```python
from build123d import *

# Parameters (mm, degrees)
F0_W     = 79.3
F0_H     = 7.4
F0_R     = 3
F1_DEPTH = 3.95
F0_R_2   = 2.499
F2_DEPTH = 2.95
F3_R     = 3.69999


# Not quite as in the source:
# - a fillet or chamfer is up to 0.001 mm smaller than in the source, because OpenCascade refuses the exact size


with BuildPart() as f1:
    # F0 (on Front) → F1 (new body, symmetric)
    with BuildSketch(Plane.XZ):
        with Locations((-4, 0)):
            Rectangle(F0_W, F0_H)
        with Locations((-40, 0)):
            Circle(F0_R, mode=Mode.SUBTRACT)
        with Locations((-32, 0)):
            Circle(F0_R, mode=Mode.SUBTRACT)
        with Locations((-24, 0)):
            Circle(F0_R, mode=Mode.SUBTRACT)
        with Locations((-16, 0)):
            Circle(F0_R, mode=Mode.SUBTRACT)
        with Locations((-8, 0)):
            Circle(F0_R, mode=Mode.SUBTRACT)
        Circle(F0_R, mode=Mode.SUBTRACT)
        with Locations((8, 0)):
            Circle(F0_R, mode=Mode.SUBTRACT)
        with Locations((16, 0)):
            Circle(F0_R, mode=Mode.SUBTRACT)
        with Locations((24, 0)):
            Circle(F0_R, mode=Mode.SUBTRACT)
        with Locations((32, 0)):
            Circle(F0_R, mode=Mode.SUBTRACT)
    extrude(amount=F1_DEPTH, both=True)

    # F0 (on Front) → F2 (join, symmetric)
    with BuildSketch(Plane.XZ):
        with Locations((-40, 0)):
            Circle(F0_R)
        with Locations((-40, 0)):
            Circle(F0_R_2, mode=Mode.SUBTRACT)
        with Locations((-32, 0)):
            Circle(F0_R)
        with Locations((-32, 0)):
            Circle(F0_R_2, mode=Mode.SUBTRACT)
        with Locations((-24, 0)):
            Circle(F0_R)
        with Locations((-24, 0)):
            Circle(F0_R_2, mode=Mode.SUBTRACT)
        with Locations((-16, 0)):
            Circle(F0_R)
        with Locations((-16, 0)):
            Circle(F0_R_2, mode=Mode.SUBTRACT)
        with Locations((-8, 0)):
            Circle(F0_R)
        with Locations((-8, 0)):
            Circle(F0_R_2, mode=Mode.SUBTRACT)
        Circle(F0_R)
        Circle(F0_R_2, mode=Mode.SUBTRACT)
        with Locations((8, 0)):
            Circle(F0_R)
        with Locations((8, 0)):
            Circle(F0_R_2, mode=Mode.SUBTRACT)
        with Locations((16, 0)):
            Circle(F0_R)
        with Locations((16, 0)):
            Circle(F0_R_2, mode=Mode.SUBTRACT)
        with Locations((24, 0)):
            Circle(F0_R)
        with Locations((24, 0)):
            Circle(F0_R_2, mode=Mode.SUBTRACT)
        with Locations((32, 0)):
            Circle(F0_R)
        with Locations((32, 0)):
            Circle(F0_R_2, mode=Mode.SUBTRACT)
    extrude(amount=F2_DEPTH, both=True)

    # F3 (radius 3.7 in the source; OpenCascade refuses exactly that, so slightly less here)
    f3_edges = [f1.edges().sort_by_distance(p)[0] for p in [
        (-43.65, 0, 3.7),
        (35.65, 0, 3.7),
        (35.65, 0, -3.7),
        (-43.65, 0, -3.7),
    ]]
    fillet(f3_edges, radius=F3_R)


solid = f1.part
```
Read the model definition and answer for the solid it produces. Units are mm, in the model's axes. A direction names the side the tool comes from. Round coordinates to 2 decimals unless told otherwise and drop trailing zeros. Write each loop counter-clockwise with the first axis right and the second up, starting at its lowest first coordinate (ties: lowest second). Pieces come first, ordered by that corner, then holes. Notation, with made-up numbers: (-25, 89) -> (29, 89) arc R16 cw to (29, 119) -> close; hole circle Ø9 at (71, -0.75). An arc over 180 degrees is marked (long way). Answer in a Markdown table with one row per item. Add a question column.
1) Consider line 1 (Z direction, x = 0, y = -3.25); line 2 (Z direction, x = 0, y = -0.8). Determine where each line is inside the solid, lowest interval first.
2) Find section C-C, the plane x = 15. Determine the outline of the cut face in (y, z), and give its area (3 significant figures).
3) Determine the mould class of faces 1 (the face through (-4.6, -3.95, 0.1)), 2 (the face through (-42.59, -0.06, -2.59)), 3 (the face through (-3, -3.4, 0.1)) for opening direction X: pulls with the +X half, pulls with the -X half, needs draft (parallel to the pull), parting line crosses it, or undercut.
4) Given P1, Ø3, axis at x = 0, z = 0, coming from the +Y side; P2, Ø1.5, axis at y = 2.5, z = -1, coming from the +X side; P3, Ø2, axis at y = 1, z = -2, coming from the -X side; P4, Ø3, axis at x = -16.5, z = -1, coming from the +Y side, each flat-ended and moving along its own axis, determine where each tip first touches the part or whether it passes through.
5) Which of the six approach directions +Z, -Z, +X, -X, +Y, -Y give full straight-line access (tool end or side, diameter ignored) to faces 4 (the face through (-19, -3.4, 0.1)), 5 (the face through (13, 3.5, 0.1)), 6 (the face through (-4.6, 3.95, 0.1))?
6) Find section A-A, the plane x = -16. Determine the outline of the cut face in (y, z).
7) Find section B-B, the plane y = 1.75. State how many separate pieces and enclosed holes the cut face has, and give its area (3 significant figures).
Findings below:
| question | item | result |
|---|---|---|
| 1 | line 1 | -3.7 to -3, 3 to 3.7 |
| 1 | line 2 | -3.7 to -2.5, 2.5 to 3.7 |
| 2 | outline | (-3.95, -3.7) -> (3.95, -3.7) -> (3.95, -2.83) -> (2.95, -2.83) -> (2.95, -2.29) -> (-2.95, -2.29) -> (-2.95, -2.83) -> (-3.95, -2.83) -> close; (-3.95, 2.83) -> (-2.95, 2.83) -> (-2.95, 2.29) -> (2.95, 2.29) -> (2.95, 2.83) -> (3.95, 2.83) -> (3.95, 3.7) -> (-3.95, 3.7) -> close |
| 2 | area | 20.1 mm² |
| 3 | face 1 | needs draft |
| 3 | face 2 | pulls with the -X half |
| 3 | face 3 | undercut |
| 4 | P1 | through |
| 4 | P2 | x = 35.64 |
| 4 | P3 | x = -43.51 |
| 4 | P4 | y = 2.95 |
| 5 | face 4 | -Y |
| 5 | face 5 | +Y |
| 5 | face 6 | +Z, -Z, +X, -X, +Y |
| 6 | outline | (-3.95, -3.7) -> (3.95, -3.7) -> (3.95, -3) -> (2.95, -3) -> (2.95, -2.5) -> (-2.95, -2.5) -> (-2.95, -3) -> (-3.95, -3) -> close; (-3.95, 3) -> (-2.95, 3) -> (-2.95, 2.5) -> (2.95, 2.5) -> (2.95, 3) -> (3.95, 3) -> (3.95, 3.7) -> (-3.95, 3.7) -> close |
| 7 | separate pieces | 1 |
| 7 | enclosed holes | 10 |
| 7 | area | 379 mm² |
